Part model, mm, in its own coordinate system. Face numbers are marked on the shaded views. A direction names the side the tool comes from. Round coordinates to 2 decimals unless told otherwise and drop trailing zeros. Write each loop counter-clockwise with the first axis right and the second up, starting at its lowest first coordinate (ties: lowest second). Pieces come first, ordered by that corner, then holes. Notation, with made-up numbers: (29.25, -28) -> (34.25, -28) arc R18 cw to (34.25, -15) -> close; hole circle Ø10 at (11, 39.25). An arc over 180 degrees is marked (long way). Return JSON: item names as keys, results as strings. Group by question number.
(1) Saw through at A-A (x = 0). List the corners of the cut face in (y, z).
(2) Saw through at D-D (y = 31.5). List the corners of the cut face in (x, z), plus the area to 3 significant figures.
(3) Tool access for the marked faces 1 and 2: list every direction of +Z, -Z, +X, -X, +Y, -Y with a clear straight run to the whole face (end or side of a thin tool).
(4) Drill centre lines: L1, parallel to Z at x = 0, y = 3.75; L2, parallel to X at y = 37, z = 0. Where is each one in solid material? Low to high. Write a range as from..to.
(5) Mould opens along Z. For the marked faces 3, 4 and 5 say: +Z half, -Z half, draft (parallel to the pull), parting line (faces both ways), or undercut.
(6) Saw through at B-B (z = 0). List the corners of the cut face in (x, y).
(7) Drop flat-ended pins along their axis: pin 1 Ø8.5 at (x, z) = (0, -71.75) entering from -Y; pin 2 Ø2 at (x, z) = (14, -20) entering from -Y; pin 3 Ø4 at (y, z) = (6, 25.5) entering from -X; pin 4 Ø10 at (y, z) = (29, 37) entering from +X. Give the stop position or say it passes through.
(8) Saw through at C-C (x = 15). List the corners of the cut face in (y, z), plus the area to 3 significant figures.
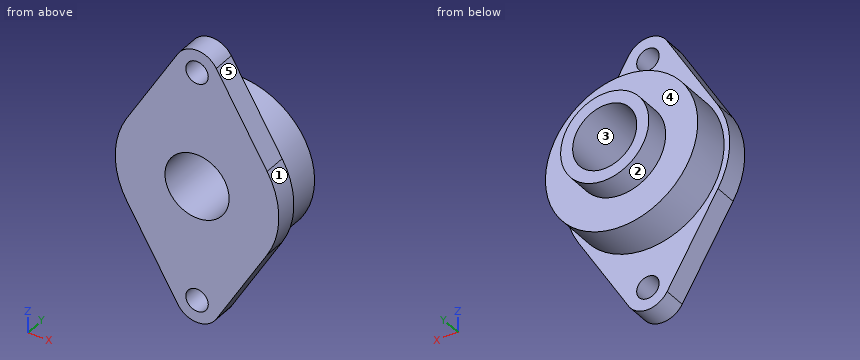
from build123d import *

# Parameters (mm, degrees)
SKETCH1_R           = 14
SKETCH1_R_2         = 7
SKETCH1_R_3         = 51
SKETCH1_R_4         = 20
BOSS_EXTRUDE1_DEPTH = 14
SKETCH2_R           = 47.5
SKETCH2_R_2         = 20
BOSS_EXTRUDE2_DEPTH = 24.5
SKETCH3_R           = 27.5
SKETCH3_R_2         = 20
BOSS_EXTRUDE3_DEPTH = 15.7


with BuildPart() as part:
    # Sketch1 → Boss-Extrude1 (new body)
    with BuildSketch(Plane(origin=(0, 0, 0), x_dir=(1, 0, 0), z_dir=(0, 1, 0))):
        with Locations((0, 71.75)):
            Circle(SKETCH1_R)
        with Locations((0, 71.75)):
            Circle(SKETCH1_R_2, mode=Mode.SUBTRACT)
        with BuildLine():
            Line((43.695861674, 26.299651568), (11.99494242, 78.969512195))
            ThreePointArc((11.99494242, 78.969512195), (13.489425375, 75.496385332), (14, 71.75))
            ThreePointArc((14, 71.75), (-3.746385332, 58.260574625), (-11.99494242, 78.969512195))
            Line((-11.99494242, 78.969512195), (-43.695861674, 26.299651568))
            ThreePointArc((-43.695861674, 26.299651568), (0, 51), (43.695861674, 26.299651568))
        make_face()
        with BuildLine():
            ThreePointArc((43.695861674, -26.299651568), (0, -51), (-43.695861674, -26.299651568))
            Line((-43.695861674, -26.299651568), (-11.99494242, -78.969512195))
            ThreePointArc((-11.99494242, -78.969512195), (-3.746385332, -58.260574625), (14, -71.75))
            ThreePointArc((14, -71.75), (13.489425375, -75.496385332), (11.99494242, -78.969512195))
            Line((11.99494242, -78.969512195), (43.695861674, -26.299651568))
        make_face()
        with Locations((0, -71.75)):
            Circle(SKETCH1_R)
        with Locations((0, -71.75)):
            Circle(SKETCH1_R_2, mode=Mode.SUBTRACT)
        Circle(SKETCH1_R_3)
        Circle(SKETCH1_R_4, mode=Mode.SUBTRACT)
    extrude(amount=BOSS_EXTRUDE1_DEPTH)

    # Sketch2 → Boss-Extrude2 (add)
    with BuildSketch(Plane(origin=(0, 14, 0), x_dir=(1, 0, 0), z_dir=(0, 1, 0))):
        Circle(SKETCH2_R)
        Circle(SKETCH2_R_2, mode=Mode.SUBTRACT)
    extrude(amount=BOSS_EXTRUDE2_DEPTH)

    # Sketch3 → Boss-Extrude3 (add)
    with BuildSketch(Plane(origin=(0, 38.5, 0), x_dir=(1, 0, 0), z_dir=(0, 1, 0))):
        Circle(SKETCH3_R)
        Circle(SKETCH3_R_2, mode=Mode.SUBTRACT)
    extrude(amount=BOSS_EXTRUDE3_DEPTH)


solid = part.part
Computed values:
{
 "1": {"outline": "(0, -85.75) -> (14, -85.75) -> (14, -78.75) -> (0, -78.75) -> close; (0, -64.75) -> (14, -64.75) -> (14, -47.5) -> (38.5, -47.5) -> (38.5, -27.5) -> (54.2, -27.5) -> (54.2, -20) -> (0, -20) -> close; (0, 20) -> (54.2, 20) -> (54.2, 27.5) -> (38.5, 27.5) -> (38.5, 47.5) -> (14, 47.5) -> (14, 64.75) -> (0, 64.75) -> close; (0, 78.75) -> (14, 78.75) -> (14, 85.75) -> (0, 85.75) -> close"},
 "2": {"outline": "circle Ø95 at (0, 0); hole circle Ø40 at (0, 0)", "area": "5,830 mm2"},
 "3": {"face 1": "+X, +Y, -Y", "face 2": "+Y"},
 "4": {"L1": "-85.75..-78.75, -64.75..-20, 20..64.75, 78.75..85.75", "L2": "-47.5..-20, 20..47.5"},
 "5": {"face 3": "undercut", "face 4": "draft", "face 5": "+Z half"},
 "6": {"outline": "(-51, 0) -> (-20, 0) -> (-20, 54.2) -> (-27.5, 54.2) -> (-27.5, 38.5) -> (-47.5, 38.5) -> (-47.5, 14) -> (-51, 14) -> close; (20, 0) -> (51, 0) -> (51, 14) -> (47.5, 14) -> (47.5, 38.5) -> (27.5, 38.5) -> (27.5, 54.2) -> (20, 54.2) -> close"},
 "7": {"pin 1": "through", "pin 2": "y = 0", "pin 3": "x = -45.26", "pin 4": "x = 35.1"},
 "8": {"outline": "(0, -73.98) -> (14, -73.98) -> (14, -45.07) -> (38.5, -45.07) -> (38.5, -23.05) -> (54.2, -23.05) -> (54.2, -13.23) -> (0, -13.23) -> close; (0, 13.23) -> (54.2, 13.23) -> (54.2, 23.05) -> (38.5, 23.05) -> (38.5, 45.07) -> (14, 45.07) -> (14, 73.98) -> (0, 73.98) -> close", "area": "3,570 mm2"}
}
